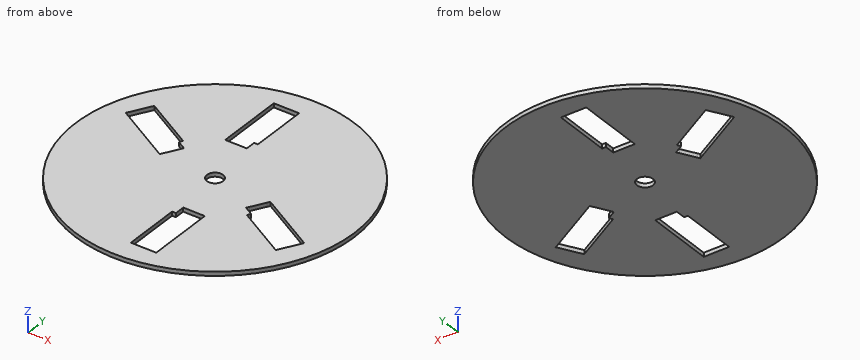
```python
from build123d import *

# Parameters (mm, degrees)
SKETCH1_R           = 110
SKETCH1_R_2         = 6.35
BOSS_EXTRUDE1_DEPTH = 1.5875


with BuildPart() as part:
    # Sketch1 → Boss-Extrude1 (new body, symmetric)
    with BuildSketch(Plane.XY):
        Circle(SKETCH1_R)
        Circle(SKETCH1_R_2, mode=Mode.SUBTRACT)
        Polygon((-6.35, 40), (-3.85, 40), (-3.85, 48), (-0.85, 48), (-0.85, 93), (-20.85, 93), (-20.85, 40), (-18.35, 40), align=None, mode=Mode.SUBTRACT)
        Polygon((6.35, -40), (3.85, -40), (3.85, -48), (0.85, -48), (0.85, -93), (20.85, -93), (20.85, -40), (18.35, -40), align=None, mode=Mode.SUBTRACT)
        Polygon((37.816016151, -14.500738686), (36.566016151, -16.665802195), (43.494219382, -20.665802195), (41.994219382, -23.263878407), (80.965362552, -45.763878407), (90.965362552, -28.443370331), (45.066016151, -1.943370331), (43.816016151, -4.108433841), align=None, mode=Mode.SUBTRACT)
        Polygon((-37.816016151, 14.500738686), (-36.566016151, 16.665802195), (-43.494219382, 20.665802195), (-41.994219382, 23.263878407), (-80.965362552, 45.763878407), (-90.965362552, 28.443370331), (-45.066016151, 1.943370331), (-43.816016151, 4.108433841), align=None, mode=Mode.SUBTRACT)
    extrude(amount=BOSS_EXTRUDE1_DEPTH, both=True)


solid = part.part
```
Geometry check sheet. Reference: the model listing, model coordinates, mm. Give positions to 0.01 mm unless a question says otherwise; leave off trailing zeros. Loops run counter-clockwise (first coordinate to the right, second up) from the corner with the lowest first, then second, coordinate; pieces in that order, holes last. Notation, with made-up numbers: M -9,29 L 2,29 A25 cw 2,57 Z; hole C 74,72 d9. An arc over 180 degrees is marked long. Write item = value, one per line.
(1) Sectioned sample at D-D, the plane x = -28.5. Record the cut outline in (y, z).
Answer below:
outline = M -106.24,-1.59 L 106.24,-1.59 L 106.24,1.59 L -106.24,1.59 Z
(2) Gauge pin test, flat ends, axial feed: pin 1 Ø1.6 at (x, z) = (12.5, 0) entering from -Y; pin 2 Ø1.5 at (x, z) = (-3, 0) entering from +Y; pin 3 Ø1.6 at (y, z) = (-72, 0.5) entering from +X. Record the tip position at first contact, or that the pin passes through.
Answer below:
pin_1 = -109.38
pin_2 = 109.98
pin_3 = 83.85
(3) Sectioned sample at C-C, the plane y = 50.5. Record the cut outline in (x, z).
Answer below:
outline = M -97.72,-1.59 L -20.85,-1.59 L -20.85,1.59 L -97.72,1.59 Z; M -0.85,-1.59 L 97.72,-1.59 L 97.72,1.59 L -0.85,1.59 Z
(4) Sectioned sample at B-B, the plane z = 0.7. Record the cut outline in (x, y).
Answer below:
outline = C 0,0 d220; hole M -90.97,28.44 L -45.07,1.94 L -36.57,16.67 L -43.49,20.67 L -41.99,23.26 L -80.97,45.76 Z; hole M -20.85,40 L -3.85,40 L -3.85,48 L -0.85,48 L -0.85,93 L -20.85,93 Z; hole C 0,0 d12.7; hole M 0.85,-93 L 20.85,-93 L 20.85,-40 L 3.85,-40 L 3.85,-48 L 0.85,-48 Z; hole M 36.57,-16.67 L 43.49,-20.67 L 41.99,-23.26 L 80.97,-45.76 L 90.97,-28.44 L 45.07,-1.94 Z
(5) Sectioned sample at A-A, the plane x = 87. Record the cut outline in (y, z), plus the area to 3 significant figures.
Answer below:
outline = M -67.31,-1.59 L -35.31,-1.59 L -35.31,1.59 L -67.31,1.59 Z; M -26.15,-1.59 L 67.31,-1.59 L 67.31,1.59 L -26.15,1.59 Z
area = 398 mm2
(6) Material ranges on line 1 (Y direction, x = 0, z = 0.9); line 2 (Y direction, x = -48, z = 0.45); line 3 (X direction, y = -86, z = -1.1), recorded low to high. Write a range as [from, to].
Answer below:
line_1 = [-110, -6.35], [6.35, 110]
line_2 = [-98.97, 3.64], [26.73, 98.97]
line_3 = [-68.59, 0.85], [20.85, 68.59]
